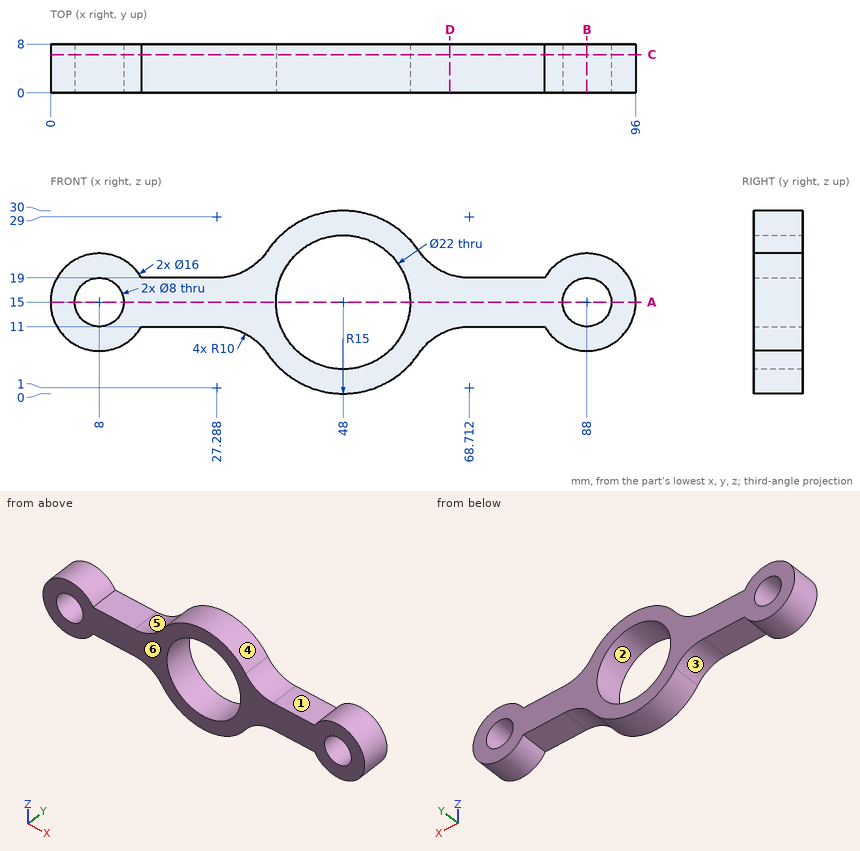
Verification items for this drawing (mm, ordinates from the low corner). A direction names the side the tool comes from. Give positions to 0.01 mm unless a question says otherwise; leave off trailing zeros. Loops run counter-clockwise (first coordinate to the right, second up) from the corner with the lowest first, then second, coordinate; pieces in that order, holes last. Notation, with made-up numbers: M 70,73.25 L 87,73.25 A32 cw 87,101.25 Z; hole C 16,-38.75 d4. An arc over 180 degrees is marked long. Answer as a JSON object with one key per item and string values. Group by question number.
Item 1: Sectioned sample at A-A on z = 15. Record the boundary of the cut face in (x, y).
Item 2: Sectioned sample at C-C on y = 6.25. Record the boundary of the cut face in (x, z).
Item 3: Sectioned sample at D-D on x = 65.5. Record the boundary of the cut face in (y, z), plus the area to 3 significant figures.
Item 4: Sectioned sample at B-B on x = 88. Record the boundary of the cut face in (y, z), plus the area to 3 significant figures.
Item 5: Gauge pin test, flat ends, axial feed: pin 1 (8 mm diameter, centred on x = 47.5, z = 20.5, fed in from +Y); pin 2 (4 mm diameter, centred on x = 22, y = 2, fed in from +Z); pin 3 (3 mm diameter, centred on x = 58.5, z = 3, fed in from +Y). Record the tip position at first contact, or that the pin passes through.
Item 6: Mould release check, pull along X, two halves, no side actions. Record for the marked faces 4, 5 and 6: pulls with the +X half, pulls with the -X half, needs draft (parallel to the pull), parting line crosses it, or undercut.
Item 7: Access from +Z, -Z, +X, -X, +Y, -Y to the whole of each face (thin tool, end or side, straight path). Record for the marked faces 1, 2 and 3.
Item 8: Material ranges on L1, parallel to X at y = 2.25, z = 15; L2, parallel to X at y = 2.25, z = 16.5; L3, parallel to Z at x = 68.5, y = 2, recorded low to high.
Findings below:
{
 "1": {"outline": "M 0,0 L 4,0 L 4,8 L 0,8 Z; M 12,0 L 37,0 L 37,8 L 12,8 Z; M 59,0 L 84,0 L 84,8 L 59,8 Z; M 92,0 L 96,0 L 96,8 L 92,8 Z"},
 "2": {"outline": "M 14.93,11 L 27.29,11 A10 cw 35.57,6.6 A15 ccw 60.43,6.6 A10 cw 68.71,11 L 81.07,11 A8 ccw long 81.07,19 L 68.71,19 A10 cw 60.43,23.4 A15 ccw 35.57,23.4 A10 cw 27.29,19 L 14.93,19 A8 ccw long Z; hole C 8,15 d8; hole C 48,15 d22; hole C 88,15 d8"},
 "3": {"outline": "M 0,10.47 L 8,10.47 L 8,19.53 L 0,19.53 Z", "area": "72.5 mm2"},
 "4": {"outline": "M 0,7 L 8,7 L 8,11 L 0,11 Z; M 0,19 L 8,19 L 8,23 L 0,23 Z", "area": "64.0 mm2"},
 "5": {"pin 1": "through", "pin 2": "z = 19", "pin 3": "y = 8"},
 "6": {"face 4": "parting line crosses it", "face 5": "undercut", "face 6": "needs draft"},
 "7": {"face 1": "+Z, +Y, -Y", "face 2": "+Y, -Y", "face 3": "-Z, +Y, -Y"},
 "8": {"L1": "0 to 4, 12 to 37, 59 to 84, 92 to 96", "L2": "0.14 to 4.29, 11.71 to 37.1, 58.9 to 84.29, 91.71 to 95.86", "L3": "11 to 19"}
}
